Part model, mm, in its own coordinate system. A direction names the side the tool comes from. Coordinates: 2 decimals unless noted, no trailing zeros. Loops run counter-clockwise (first coordinate to the right, second up) from the corner with the lowest first, then second, coordinate; pieces in that order, holes last.
```python
from build123d import *

# Parameters (mm, degrees)
F0_R        = 1.5875
F0_R_2      = 4.7625
F1_DEPTH    = 6.35
F2_T1_DEPTH = 6.35
F3_R        = 25.6632962838


# Not quite as in the source:
# - a fillet or chamfer that OpenCascade refuses, or shapes differently, is made with other operations: its cross-section is extruded or revolved along the edge and cut away or added
# - a length typed as a fraction of an inch, garbled in the dataset ("3 / 203.2 mm" for 3/8 in), is restored


with BuildPart() as f1:
    # F0 (on Top) → F1 (new body)
    with BuildSketch(Plane.XY):
        with BuildLine():
            Line((25.7948291982, 22.225), (38.4948291982, 22.225))
            Line((38.4948291982, 22.225), (32.1448291982, 11.2264773719))
            Line((32.1448291982, 11.2264773719), (65.1403970824, 30.2764773719))
            ThreePointArc((65.1403970824, 30.2764773719), (67.4646583964, 38.950738686), (58.7903970824, 41.275))
            Line((58.7903970824, 41.275), (25.7948291982, 22.225))
        make_face()
        with Locations((61.9653970824, 35.775738686)):
            Circle(F0_R, mode=Mode.SUBTRACT)
        with BuildLine():
            Line((32.1448291982, 11.2264773719), (38.4948291982, 22.225))
            Line((38.4948291982, 22.225), (25.7948291982, 22.225))
            Line((25.7948291982, 22.225), (20.8585659862, 22.225))
            ThreePointArc((20.8585659862, 22.225), (26.3964543073, 15.24), (29.6766975922, 6.9515480306))
            Line((29.6766975922, 6.9515480306), (32.1448291982, 11.2264773719))
        make_face()
        with Locations((30.7958633586, 17.78)):
            Circle(F0_R, mode=Mode.SUBTRACT)
        with BuildLine():
            ThreePointArc((30.48, 0), (30.2785084062, 3.4989039276), (29.6766975922, 6.9515480306))
            Line((29.6766975922, 6.9515480306), (21.0222935562, -8.0383194689))
            ThreePointArc((21.0222935562, -8.0383194689), (21.2004099791, -8.7721955059), (21.2602839421, -9.525))
            ThreePointArc((21.2602839421, -9.525), (20.1939753076, -12.5282608344), (17.472535642, -14.1866805311))
            Line((17.472535642, -14.1866805311), (8.818131606, -29.1765480305))
            ThreePointArc((8.818131606, -29.1765480305), (24.4725055047, -18.1693938898), (30.48, 0))
        make_face()
        with BuildLine():
            Line((21.0222935562, -8.0383194689), (29.6766975922, 6.9515480306))
            ThreePointArc((29.6766975922, 6.9515480306), (26.3964543073, 15.24), (20.8585659862, 22.225))
            Line((20.8585659862, 22.225), (3.5497579143, 22.225))
            ThreePointArc((3.5497579143, 22.225), (4.4489958596, 20.7493652025), (4.7625, 19.05))
            ThreePointArc((4.7625, 19.05), (-1.6993652025, 14.6010041404), (-3.5497579143, 22.225))
            Line((-3.5497579143, 22.225), (-20.8585659862, 22.225))
            ThreePointArc((-20.8585659862, 22.225), (-26.3964543073, 15.24), (-29.6766975922, 6.9515480306))
            Line((-29.6766975922, 6.9515480306), (-21.0222935562, -8.0383194689))
            ThreePointArc((-21.0222935562, -8.0383194689), (-15.744979448, -4.822373963), (-11.7352839421, -9.525))
            ThreePointArc((-11.7352839421, -9.525), (-13.4945231077, -13.2211913655), (-17.472535642, -14.1866805311))
            Line((-17.472535642, -14.1866805311), (-8.818131606, -29.1765480305))
            ThreePointArc((-8.818131606, -29.1765480305), (0, -30.48), (8.818131606, -29.1765480305))
            Line((8.818131606, -29.1765480305), (17.472535642, -14.1866805311))
            ThreePointArc((17.472535642, -14.1866805311), (12.3733379566, -7.14375), (21.0222935562, -8.0383194689))
        make_face()
        with Locations((0, -25.4)):
            Circle(F0_R_2, mode=Mode.SUBTRACT)
        with Locations((-21.9970452561, 12.7)):
            Circle(F0_R_2, mode=Mode.SUBTRACT)
        Circle(F0_R_2, mode=Mode.SUBTRACT)
        with Locations((21.9970452561, 12.7)):
            Circle(F0_R_2, mode=Mode.SUBTRACT)
        with BuildLine():
            Line((3.5497579143, 22.225), (20.8585659862, 22.225))
            ThreePointArc((20.8585659862, 22.225), (0, 30.48), (-20.8585659862, 22.225))
            Line((-20.8585659862, 22.225), (-3.5497579143, 22.225))
            ThreePointArc((-3.5497579143, 22.225), (0, 23.8125), (3.5497579143, 22.225))
        make_face()
        with BuildLine():
            ThreePointArc((-29.6766975922, 6.9515480306), (-26.3964543073, 15.24), (-20.8585659862, 22.225))
            Line((-20.8585659862, 22.225), (-25.7948291982, 22.225))
            Line((-25.7948291982, 22.225), (-38.4948291982, 22.225))
            Line((-38.4948291982, 22.225), (-32.1448291982, 11.2264773719))
            Line((-32.1448291982, 11.2264773719), (-29.6766975922, 6.9515480306))
        make_face()
        with Locations((-30.7958633586, 17.78)):
            Circle(F0_R, mode=Mode.SUBTRACT)
        with BuildLine():
            Line((6.35, -33.4514773719), (8.818131606, -29.1765480305))
            ThreePointArc((8.818131606, -29.1765480305), (0, -30.48), (-8.818131606, -29.1765480305))
            Line((-8.818131606, -29.1765480305), (-6.35, -33.4514773719))
            Line((-6.35, -33.4514773719), (0, -44.45))
            Line((0, -44.45), (6.35, -33.4514773719))
        make_face()
        with Locations((0, -35.56)):
            Circle(F0_R, mode=Mode.SUBTRACT)
        with BuildLine():
            Line((-38.4948291982, 22.225), (-25.7948291982, 22.225))
            Line((-25.7948291982, 22.225), (-58.7903970824, 41.275))
            ThreePointArc((-58.7903970824, 41.275), (-67.4646583964, 38.950738686), (-65.1403970824, 30.2764773719))
            Line((-65.1403970824, 30.2764773719), (-32.1448291982, 11.2264773719))
            Line((-32.1448291982, 11.2264773719), (-38.4948291982, 22.225))
        make_face()
        with Locations((-61.9653970824, 35.775738686)):
            Circle(F0_R, mode=Mode.SUBTRACT)
        with BuildLine():
            Line((-21.0222935562, -8.0383194689), (-29.6766975922, 6.9515480306))
            ThreePointArc((-29.6766975922, 6.9515480306), (-26.3964543073, -15.24), (-8.818131606, -29.1765480305))
            Line((-8.818131606, -29.1765480305), (-17.472535642, -14.1866805311))
            ThreePointArc((-17.472535642, -14.1866805311), (-20.6222299276, -11.90625), (-21.0222935562, -8.0383194689))
        make_face()
        with BuildLine():
            Line((6.35, -71.5514773719), (6.35, -33.4514773719))
            Line((6.35, -33.4514773719), (0, -44.45))
            Line((0, -44.45), (-6.35, -33.4514773719))
            Line((-6.35, -33.4514773719), (-6.35, -71.5514773719))
            ThreePointArc((-6.35, -71.5514773719), (0, -77.9014773719), (6.35, -71.5514773719))
        make_face()
        with Locations((0, -71.5514773719)):
            Circle(F0_R, mode=Mode.SUBTRACT)
    extrude(amount=F1_DEPTH)

    # F2: fillet of radius 50.8 on 6 edges, made by hand

    # F2_s2 → F2_t1 (join)
    with BuildSketch(Plane.XY):
        with BuildLine():
            ThreePointArc((29.6766975922, 6.9515480306), (35.4424077678, 12.4134665997), (41.9889550232, 16.9099860669))
            Line((41.9889550232, 16.9099860669), (32.1448291982, 11.2264773719))
            Line((32.1448291982, 11.2264773719), (29.6766975922, 6.9515480306))
        make_face()
        with BuildLine():
            ThreePointArc((35.6389550232, 27.908508695), (28.4715813083, 24.4872921983), (20.8585659862, 22.225))
            Line((20.8585659862, 22.225), (25.7948291982, 22.225))
            Line((25.7948291982, 22.225), (35.6389550232, 27.908508695))
        make_face()
        with BuildLine():
            ThreePointArc((-20.8585659862, 22.225), (-28.4715813083, 24.4872921983), (-35.6389550232, 27.908508695))
            Line((-35.6389550232, 27.908508695), (-25.7948291982, 22.225))
            Line((-25.7948291982, 22.225), (-20.8585659862, 22.225))
        make_face()
        with BuildLine():
            ThreePointArc((-41.9889550232, 16.9099860669), (-35.4424077678, 12.4134665997), (-29.6766975922, 6.9515480306))
            Line((-29.6766975922, 6.9515480306), (-32.1448291982, 11.2264773719))
            Line((-32.1448291982, 11.2264773719), (-41.9889550232, 16.9099860669))
        make_face()
        with BuildLine():
            ThreePointArc((-8.818131606, -29.1765480305), (-6.9708264595, -36.9007587981), (-6.35, -44.8184947619))
            Line((-6.35, -44.8184947619), (-6.35, -33.4514773719))
            Line((-6.35, -33.4514773719), (-8.818131606, -29.1765480305))
        make_face()
        with BuildLine():
            ThreePointArc((6.35, -44.8184947619), (6.9708264595, -36.9007587981), (8.818131606, -29.1765480305))
            Line((8.818131606, -29.1765480305), (6.35, -33.4514773719))
            Line((6.35, -33.4514773719), (6.35, -44.8184947619))
        make_face()
    extrude(amount=F2_T1_DEPTH)

    # F3
    f3_edges = [f1.edges().sort_by_distance(p)[0] for p in [
        (-29.676698, 6.951548, 3.175),
        (-8.818132, -29.176548, 3.175),
        (8.818132, -29.176548, 3.175),
        (29.676698, 6.951548, 3.175),
        (20.858566, 22.225, 3.175),
        (-20.858566, 22.225, 3.175),
    ]]
    fillet(f3_edges, radius=F3_R)


solid = f1.part
```
Q1. Probe line 1 (Y direction, x = 0, z = 3.25); line 2 (X direction, y = -7, z = 5.5); line 3 (X direction, y = 16, z = 3). List the from-to ranges inside material, lowest first.
Q2. Saw through at B-B (y = 12.7). Count the separate pieces of the cut face and the enclosed holes in it, plus the area to 3 significant figures.
Q3. Saw through at D-D (x = -54). List the corners of the cut face in (y, z).
Q4. Drop flat-ended pins along their axis: P1, Ø4, axis at x = 61.97, y = 35.78, coming from the +Z side; P2, Ø7.5, axis at x = -22, y = 12.7, coming from the +Z side; P3, Ø1.5, axis at y = 3.5, z = 4, coming from the +X side. Give the stop position or say it passes through.
Q5. Tool access for faces 1 (the cylindrical face through (-26.49, -15.08, 3.13)), 2 (the flat face through (-47.625, 34.829, 3.131)): list every direction of +Z, -Z, +X, -X, +Y, -Y with a clear straight run to the whole face (end or side of a thin tool).
Q6. Mould opens along X. For faces 3 (the cylindrical face through (-0.207, -69.977, 3.131)), 4 (the flat face through (-6.35, -59, 3)), 5 (the flat face through (-5, 0, 0)), 6 (the cylindrical face through (18.22, 9.8, 3.13)) say: released by +X, released by -X, zero draft, split by the parting line, or undercut.
Q7. Saw through at A-A (x = 0). List the corners of the cut face in (y, z).
Checked values:
1. line 1: y = -77.9 to -73.14, -69.96 to -37.15, -33.97 to -30.16, -20.64 to -4.76, 4.76 to 14.29, 23.81 to 30.48
1. line 2: x = -29.67 to -20.54, -12.46 to 12.46, 20.54 to 29.67
1. line 3: x = -40.73 to -25.43, -18.56 to -3.66, 3.66 to 18.56, 25.43 to 40.73
2. separate pieces: 3
2. enclosed holes: 0
2. area: 350 mm2
3. outline: (23.84, 0) - (38.51, 0) - (38.51, 6.35) - (23.84, 6.35) - close
4. P1: stops at z = 6.35
4. P2: passes through
4. P3: stops at x = 31.88
5. face 1: +Z, -Z, -X, -Y
5. face 2: +Z, -Z, +Y
6. face 3: undercut
6. face 4: released by -X
6. face 5: zero draft
6. face 6: undercut
7. outline: (-77.9, 0) - (-73.14, 0) - (-73.14, 6.35) - (-77.9, 6.35) - close; (-69.96, 0) - (-37.15, 0) - (-37.15, 6.35) - (-69.96, 6.35) - close; (-33.97, 0) - (-30.16, 0) - (-30.16, 6.35) - (-33.97, 6.35) - close; (-20.64, 0) - (-4.76, 0) - (-4.76, 6.35) - (-20.64, 6.35) - close; (4.76, 0) - (14.29, 0) - (14.29, 6.35) - (4.76, 6.35) - close; (23.81, 0) - (30.48, 0) - (30.48, 6.35) - (23.81, 6.35) - close
